Could you check a few things on this model? Use its own coordinates, in mm. Give positions to 0.01 mm unless a question says otherwise; leave off trailing zeros. Loops run counter-clockwise (first coordinate to the right, second up) from the corner with the lowest first, then second, coordinate; pieces in that order, holes last. Notation, with made-up numbers: M 11,0 L 50,0 A21 cw 50,39 Z; hole C -23,44 d8. An arc over 180 degrees is marked long. Answer in a Markdown table with one row per item. Add a question column.
1. I'm going to push flat-ended pins straight in: pin 1 Ø1.5 at (y, z) = (-9.5, 3) entering from +X; pin 2 Ø2 at (y, z) = (8.5, 0.5) entering from -X; pin 3 Ø2.5 at (x, z) = (30, 1.5) entering from -Y. Where does each tip first touch, or does it pass through?
2. I need wall thicknesses on line 1 along X through (y, z) = (-8, 1.35); line 2 along Y through (x, z) = (-53, 4.25); line 3 along X through (y, z) = (4.5, 1.7). Which ranges of each line are inside material? Lowest first, please. Write a range as from..to.
3. If we section it at C-C on z = 1.7: List the corners of the cut face in (x, y) for me, then the cut area to 3 significant figures.
4. If we section it at A-A on y = -8.5: List the corners of the cut face in (x, z) for me.
5. If we section it at B-B on y = 12.5: List the corners of the cut face in (x, z) for me, then the cut area to 3 significant figures.
6. If we section it at D-D on x = 22: List the corners of the cut face in (y, z) for me, then the cut area to 3 significant figures.
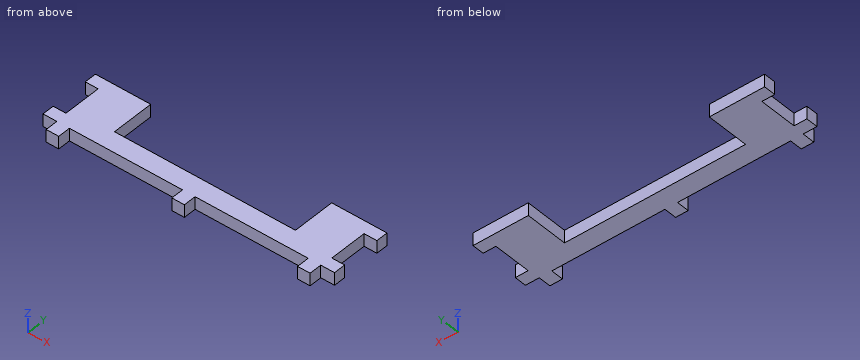
```python
from build123d import *

# Parameters (mm, degrees)
SKETCH1_W           = 116
SKETCH1_H           = 12.3
BOSS_EXTRUDE1_DEPTH = 5
SKETCH2_W           = 5
SKETCH2_H           = 5
BOSS_EXTRUDE2_DEPTH = 5
SKETCH3_W           = 72
SKETCH3_H           = 5
CUT_EXTRUDE1_DEPTH  = 17
SKETCH4_W           = 5
SKETCH4_H           = 5
BOSS_EXTRUDE3_DEPTH = 5
SKETCH5_W           = 5
SKETCH5_H           = 15.1
CUT_EXTRUDE2_DEPTH  = 5.1


with BuildPart() as part:
    # Sketch1 → Boss-Extrude1 (new body)
    with BuildSketch(Plane.XY):
        Rectangle(SKETCH1_W, SKETCH1_H)
    extrude(amount=BOSS_EXTRUDE1_DEPTH)

    # Mirror1: part across plane


with BuildPart() as part_1:
    add(part.part)
    add(part.part.mirror(Plane(origin=(-58, 6.15, 5), x_dir=(0, 0, 1), z_dir=(0, -1, 0))))

    # Sketch2 → Boss-Extrude2 (add)
    with BuildSketch(Plane.XZ.offset(6.15)):
        with Locations((-50, 2.5)):
            Rectangle(SKETCH2_W, SKETCH2_H)
        with Locations((50, 2.5)):
            Rectangle(SKETCH2_W, SKETCH2_H)
    extrude(amount=BOSS_EXTRUDE2_DEPTH)

    # Sketch3 → Cut-Extrude1 (cut)
    with BuildSketch(Plane(origin=(0, 18.45, 0), x_dir=(1, 0, 0), z_dir=(0, 1, 0))):
        with Locations((0, -2.5)):
            Rectangle(SKETCH3_W, SKETCH3_H)
    extrude(amount=-CUT_EXTRUDE1_DEPTH, mode=Mode.SUBTRACT)

    # Sketch4 → Boss-Extrude3 (add)
    with BuildSketch(Plane.XZ.offset(6.15)):
        with Locations((0, 2.5)):
            Rectangle(SKETCH4_W, SKETCH4_H)
    extrude(amount=BOSS_EXTRUDE3_DEPTH)

    # Sketch5 → Cut-Extrude2 (cut)
    with BuildSketch(Plane.ZY.offset(58)):
        with Locations((2.5, 6.15)):
            Rectangle(SKETCH5_W, SKETCH5_H)
    cut_extrude2 = extrude(amount=-CUT_EXTRUDE2_DEPTH, mode=Mode.SUBTRACT)

    # Mirror2: Cut-Extrude2 across plane
    add(cut_extrude2.mirror(Plane(origin=(0, 0, 0), x_dir=(0, 0, 1), z_dir=(1, 0, 0))), mode=Mode.SUBTRACT)


solid = part_1.part
```
Results:
| question | item | result |
|---|---|---|
| 1 | pin 1 | x = 52.5 |
| 1 | pin 2 | x = -52.9 |
| 1 | pin 3 | y = -6.15 |
| 2 | line 1 | -52.5..-47.5, -2.5..2.5, 47.5..52.5 |
| 2 | line 2 | -6.15..-1.4, 13.7..18.45 |
| 2 | line 3 | -52.9..-36, 36..52.9 |
| 3 | outline | M -58,-6.15 L -52.5,-6.15 L -52.5,-11.15 L -47.5,-11.15 L -47.5,-6.15 L -2.5,-6.15 L -2.5,-11.15 L 2.5,-11.15 L 2.5,-6.15 L 47.5,-6.15 L 47.5,-11.15 L 52.5,-11.15 L 52.5,-6.15 L 58,-6.15 L 58,-1.4 L 52.9,-1.4 L 52.9,13.7 L 58,13.7 L 58,18.45 L 36,18.45 L 36,1.45 L -36,1.45 L -36,18.45 L -58,18.45 L -58,13.7 L -52.9,13.7 L -52.9,-1.4 L -58,-1.4 Z |
| 3 | area | 1,550 mm2 |
| 4 | outline | M -52.5,0 L -47.5,0 L -47.5,5 L -52.5,5 Z; M -2.5,0 L 2.5,0 L 2.5,5 L -2.5,5 Z; M 47.5,0 L 52.5,0 L 52.5,5 L 47.5,5 Z |
| 5 | outline | M -52.9,0 L -36,0 L -36,5 L -52.9,5 Z; M 36,0 L 52.9,0 L 52.9,5 L 36,5 Z |
| 5 | area | 169 mm2 |
| 6 | outline | M -6.15,0 L 1.45,0 L 1.45,5 L -6.15,5 Z |
| 6 | area | 38.0 mm2 |
